Here's the drawing with two shaded views (mm, measured from the low corner). I have some questions. A direction names the side the tool comes from. Round coordinates to 2 decimals unless told otherwise and drop trailing zeros. Order: outer loops, then holes, each group sorted by start corner. A loop starts at its lowest first (then second) coordinate and runs counter-clockwise, first axis right, second up.
Q1. Will these pins go through, and if not, where does the flat tip stop? P1, Ø4, axis at x = 4.5, y = 5, coming from the -Z side; P2, Ø4, axis at y = 4.5, z = 11, coming from the +X side; P3, Ø3, axis at y = 6, z = 6.5, coming from the +X side (1 decimal); P4, Ø1.5, axis at y = 13.87, z = 5.89, coming from the +X side.
Q2. For the marked faces 1, 2, 3 and 4, which set-ups out of +Z, -Z, +X, -X, +Y, -Y let a thin tool reach every point of the face, with its end or its side?
Q3. If we section it at B-B (y = 5): Please give me the cut outline in (x, z).
Q4. If we section it at D-D (z = 3.5): Please give me the cut outline in (x, y) (1 decimal).
Q5. If we section it at C-C (z = 6.25): Please give me the cut outline in (x, y) (1 decimal).
Q6. If I drill on line 1 (Y direction, x = 4.5, z = 8.4); line 2 (Y direction, x = 3.5, z = 1.75); line 3 (Z direction, x = 7, y = 3.75), over which ranges is the centre line in solid material (lowest first)?
Q7. If we section it at A-A (x = 4.5): Please give me the cut outline in (y, z).
Q8. We'd pull the mould along Y, two halves only. Please class the marked faces 5, 6 and 7: pulls with the +Y half, pulls with the -Y half, needs draft (parallel to the pull), parting line crosses it, or undercut.
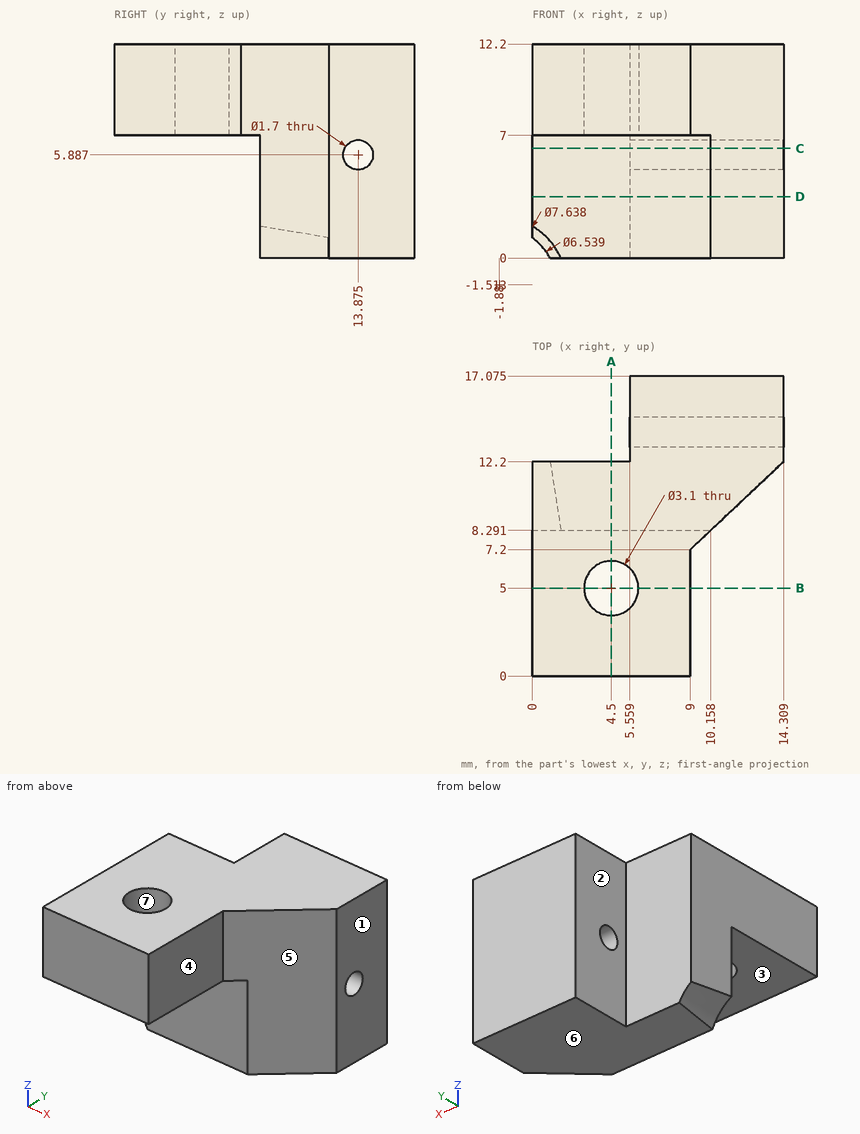
Solution:
1. P1: stops at z = 7
1. P2: stops at x = 9
1. P3: stops at x = 9.2
1. P4: passes through
2. face 1: +Z, -Z, +X, +Y, -Y
2. face 2: +Z, -Z, -X, +Y
2. face 3: -Z, +X, -X, -Y
2. face 4: +Z, -Z, +X, -Y
3. outline: (0, 7) - (2.95, 7) - (2.95, 12.2) - (0, 12.2) - close; (6.05, 7) - (9, 7) - (9, 12.2) - (6.05, 12.2) - close
4. outline: (0, 8.3) - (10.2, 8.3) - (14.3, 12.2) - (14.3, 17.1) - (5.6, 17.1) - (5.6, 12.2) - (0, 12.2) - close
5. outline: (0, 8.3) - (10.2, 8.3) - (14.3, 12.2) - (14.3, 13.1) - (5.6, 13.1) - (5.6, 12.2) - (0, 12.2) - close; (5.6, 14.6) - (14.3, 14.6) - (14.3, 17.1) - (5.6, 17.1) - close
6. line 1: y = 0 to 3.45, 6.55 to 12.2
6. line 2: y = 8.29 to 12.2
6. line 3: z = 7 to 12.2
7. outline: (0, 7) - (3.45, 7) - (3.45, 12.2) - (0, 12.2) - close; (6.55, 7) - (8.29, 7) - (8.29, 0) - (12.2, 0) - (12.2, 12.2) - (6.55, 12.2) - close
8. face 5: pulls with the -Y half
8. face 6: needs draft
8. face 7: undercut
